from build123d import *

# Parameters (mm, degrees)
F1_DEPTH = 4


with BuildPart() as f1:
    # F0 (on Top) → F1 (new body)
    with BuildSketch(Plane.XY):
        with BuildLine():
            Line((10.913862, 100.04352), (0.913862, 100.04352))
            Line((0.913862, 100.04352), (0.913862, 98.879407))
            Line((0.913862, 98.879407), (0.328076, 98.293621))
            ThreePointArc((0.328076, 98.293621), (0.761621, 96.11404), (-1.086138, 94.879407))
            ThreePointArc((-1.086138, 94.879407), (-2.955332, 96.167991), (-2.415912, 98.373295))
            Line((-2.415912, 98.373295), (-3.086138, 99.04352))
            Line((-3.086138, 99.04352), (-3.086138, 100.04352))
            Line((-3.086138, 100.04352), (-13.086138, 100.04352))
            Line((-13.086138, 100.04352), (-13.086138, 101.04352))
            Line((-13.086138, 101.04352), (-13.671924, 101.629306))
            ThreePointArc((-13.671924, 101.629306), (-15.086138, 105.04352), (-16.500351, 101.629306))
            Line((-16.500351, 101.629306), (-17.086138, 101.04352))
            Line((-17.086138, 101.04352), (-17.086138, 100.04352))
            Line((-17.086138, 100.04352), (-30.086138, 100.04352))
            Line((-30.086138, 100.04352), (-45.086138, -84.95648))
            Line((-45.086138, -84.95648), (-1.086138, -124.95648))
            Line((-1.086138, -124.95648), (42.913862, -84.95648))
            Line((42.913862, -84.95648), (27.913862, 100.04352))
            Line((27.913862, 100.04352), (14.913862, 100.04352))
            Line((14.913862, 100.04352), (10.913862, 100.04352))
        make_face()
        with BuildLine():
            Line((10.913862, 101.04352), (10.913862, 100.04352))
            Line((10.913862, 100.04352), (14.913862, 100.04352))
            Line((14.913862, 100.04352), (14.913862, 101.04352))
            Line((14.913862, 101.04352), (14.328076, 101.629306))
            ThreePointArc((14.328076, 101.629306), (12.913862, 105.04352), (11.499649, 101.629306))
            Line((11.499649, 101.629306), (10.913862, 101.04352))
        make_face()
    extrude(amount=F1_DEPTH)


solid = f1.part
For this review, take the finished solid that the model builds, in its own axes (mm). A direction names the side the tool comes from. Round coordinates to 2 decimals unless told otherwise and drop trailing zeros. Write each loop counter-clockwise with the first axis right and the second up, starting at its lowest first coordinate (ties: lowest second). Pieces come first, ordered by that corner, then holes. Notation, with made-up numbers: M 85,35 L 93,35 A10 ccw 93,49 Z; hole C 34,31.25 d4. An arc over 180 degrees is marked long. Write item = value, one per line. Start each with the question number.
(1) For line 1 along Y through (x, z) = (0.5, 0.85); line 2 along Y through (x, z) = (23.5, 1.2); line 3 along X through (y, z) = (-14.5, 0.4), list the stretches that pass through material, from the lowest coordinate up.
(2) For faces 1 (the face through (20.606, -105.236, 1.972)), 2 (the face through (22, 100.044, 2)), 3 (the face through (-8, 100.044, 2)), list the 3-axis set-ups (+Z, -Z, +X, -X, +Y, -Y) from which the entire face can be reached by the end or side of a thin tool; tool diameter is ignored.
(3) Clearance check with flat-ended pins moving along their axes: pin 1 Ø1.5 at (x, y) = (9, 47.5) entering from -Z; pin 2 Ø0.8 at (y, z) = (100.5, 2) entering from +X; pin 3 Ø1.2 at (x, z) = (-21, 1.5) entering from +Y; pin 4 Ø0.8 at (y, z) = (101, 1.5) entering from -X. State where each tip first meets the part, or that it passes through.
(4) The part is to be moulded in two halves that separate along X. For faces 4 (the face through (-23, 100.044, 2)), 5 (the face through (6, 100.044, 2)), 6 (the face through (-23.39, -104.68, 1.97)), say which applies: +X half, -X half, draft (parallel to the pull), parting line (faces both ways), or undercut.
(5) We need section B-B (x = -36). Give the boundary of the cut face in (y, z), then the cut area to 3 significant figures.
(6) We need section C-C (y = 40.5). Give the boundary of the cut face in (x, z), then the cut area to 3 significant figures.
(7) We need section A-A (z = 2.4). Give the boundary of the cut face in (x, y).
Results found:
q1.line_1 = -123.51 to 95.66, 98.1 to 98.47
q1.line_2 = -102.61 to 100.04
q1.line_3 = -39.37 to 37.2
q2.face_1 = +Z, -Z, +X, -Y
q2.face_2 = +Z, -Z, +X, +Y
q2.face_3 = +Z, -Z, +Y
q3.pin_1 = 0
q3.pin_2 = 14.91
q3.pin_3 = 100.04
q3.pin_4 = -17.09
q4.face_4 = draft
q4.face_5 = undercut
q4.face_6 = -X half
q5.outline = M -93.22,0 L 27.11,0 L 27.11,4 L -93.22,4 Z
q5.area = 481 mm²
q6.outline = M -34.91,0 L 32.74,0 L 32.74,4 L -34.91,4 Z
q6.area = 271 mm²
q7.outline = M -45.09,-84.96 L -1.09,-124.96 L 42.91,-84.96 L 27.91,100.04 L 14.91,100.04 L 14.91,101.04 L 14.33,101.63 A2 ccw long 11.5,101.63 L 10.91,101.04 L 10.91,100.04 L 0.91,100.04 L 0.91,98.88 L 0.33,98.29 A2 cw long -2.42,98.37 L -3.09,99.04 L -3.09,100.04 L -13.09,100.04 L -13.09,101.04 L -13.67,101.63 A2 ccw long -16.5,101.63 L -17.09,101.04 L -17.09,100.04 L -30.09,100.04 Z
